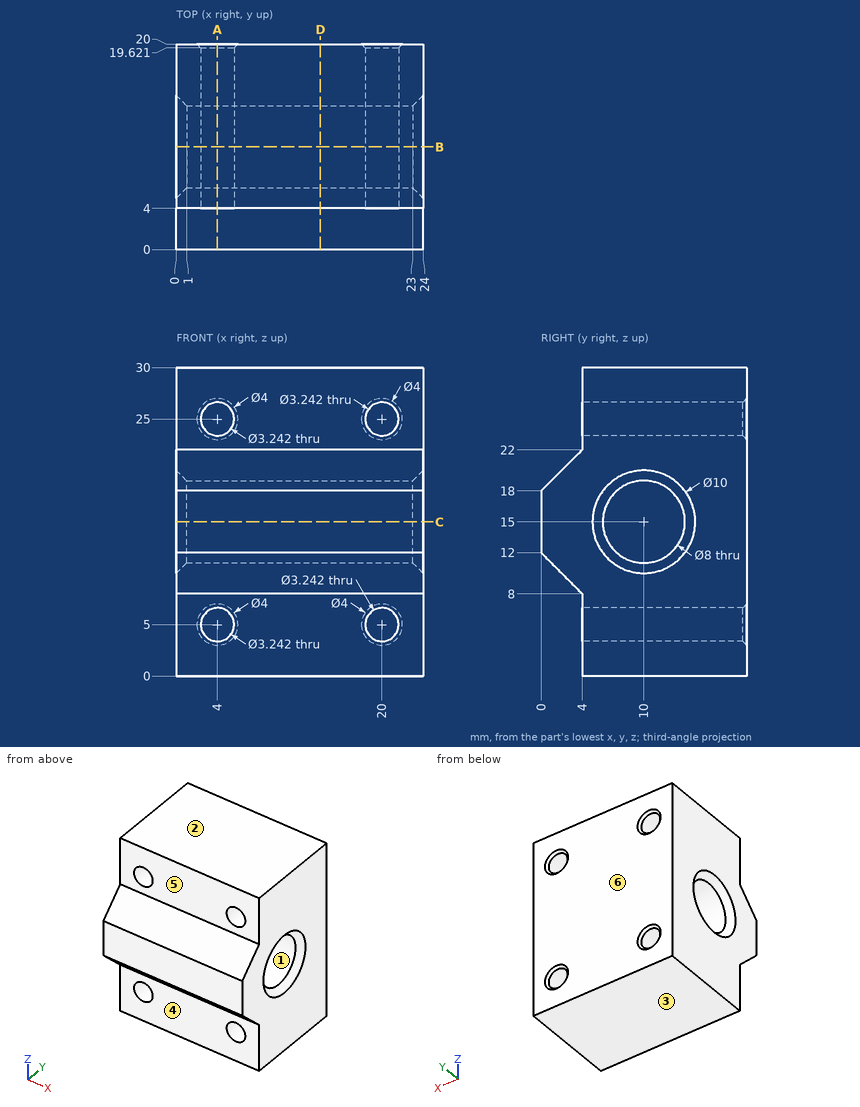
Here's the drawing with two shaded views (mm, measured from the low corner). I have some questions. A direction names the side the tool comes from. Coordinates: 2 decimals unless noted, no trailing zeros. Loops run counter-clockwise (first coordinate to the right, second up) from the corner with the lowest first, then second, coordinate; pieces in that order, holes last. Notation, with made-up numbers: M 54.25,67 L 65.25,67 A34 ccw 65.25,104 Z; hole C 39,-9.5 d1. An arc over 180 degrees is marked long. Put each result on its own line as item: value. Start each with the question number.
(1) Imagine slicing it at C-C on z = 15. List the corners of the cut face in (x, y) for me, and give its area (3 significant figures).
(2) I need wall thicknesses on probe 1 along X at (y, z) = (11.5, 25); probe 2 along Z at (x, y) = (20, 16.75); probe 3 along Z at (x, y) = (20, 8). Which ranges of each line are inside material? Lowest first, please.
(3) Imagine slicing it at B-B on y = 10. List the corners of the cut face in (x, z) for me, and give its area (3 significant figures).
(4) We'd pull the mould along Z, two halves only. Please class the marked faces 1, 2, 3 and 4: +Z half, -Z half, draft (parallel to the pull), parting line (faces both ways), or undercut.
(5) Imagine slicing it at D-D on x = 14. List the corners of the cut face in (y, z) for me, and give its area (3 significant figures).
(6) Imagine slicing it at A-A on x = 4. List the corners of the cut face in (y, z) for me.
(7) Which directions (+Z, -Z, +X, -X, +Y, -Y) give clear straight access to the entire face, cutting with the end or side of a thin tool? Please do the marked faces 5 and 6.
(8) Will these pins go through, and if not, where does the flat tip stop? pin 1 Ø4 at (x, z) = (17.5, 27) entering from -Y; pin 2 Ø12 at (x, z) = (7.5, 24.5) entering from -Y; pin 3 Ø4 at (x, z) = (20, 8.5) entering from -Y.
Worked answers:
1. outline: M 0,0 L 24,0 L 24,5 L 23,6 L 1,6 L 0,5 Z; M 0,15 L 1,14 L 23,14 L 24,15 L 24,20 L 0,20 Z
1. area: 286 mm2
2. probe 1: x = 0 to 2.38, 5.62 to 18.38, 21.62 to 24
2. probe 2: z = 0 to 3.38, 6.62 to 23.38, 26.62 to 30
2. probe 3: z = 0 to 3.38, 6.62 to 11.54, 18.46 to 23.38, 26.62 to 30
3. outline: M 0,0 L 24,0 L 24,10 L 23,11 L 1,11 L 0,10 Z; M 0,20 L 1,19 L 23,19 L 24,20 L 24,30 L 0,30 Z; hole C 4,5 d3.24; hole C 4,25 d3.24; hole C 20,5 d3.24; hole C 20,25 d3.24
3. area: 493 mm2
4. face 1: undercut
4. face 2: +Z half
4. face 3: -Z half
4. face 4: draft
5. outline: M 0,12 L 4,8 L 4,0 L 20,0 L 20,30 L 4,30 L 4,22 L 0,18 Z; hole C 10,15 d8
5. area: 470 mm2
6. outline: M 0,12 L 4,8 L 4,6.62 L 19.62,6.62 L 20,7 L 20,23 L 19.62,23.38 L 4,23.38 L 4,22 L 0,18 Z; M 4,0 L 20,0 L 20,3 L 19.62,3.38 L 4,3.38 Z; M 4,26.62 L 19.62,26.62 L 20,27 L 20,30 L 4,30 Z; hole C 10,15 d8
7. face 5: +Z, +X, -X, -Y
7. face 6: +Z, -Z, +X, -X, +Y
8. pin 1: stops at y = 4
8. pin 2: stops at y = 0.5
8. pin 3: stops at y = 1.5
